from build123d import *

# Parameters (mm, degrees)
BOSS_EXTRUDE1_DEPTH = 30
SKETCH2_R           = 1.5
CUT_EXTRUDE1_DEPTH  = 12
SKETCH3_R           = 1.5
BOSS_EXTRUDE2_DEPTH = 6


with BuildPart() as part:
    # Sketch1 → Boss-Extrude1 (new body)
    with BuildSketch(Plane(origin=(0, 0, 0), x_dir=(1, 0, 0), z_dir=(0, 1, 0))):
        Polygon((3.175426481, 0), (1.58771324, 2.75), (-1.58771324, 2.75), (-3.175426481, 0), (-1.58771324, -2.75), (1.58771324, -2.75), align=None)
    extrude(amount=BOSS_EXTRUDE1_DEPTH)

    # Sketch2 → Cut-Extrude1 (cut)
    with BuildSketch(Plane(origin=(0, 30, 0), x_dir=(1, 0, 0), z_dir=(0, 1, 0))):
        with Locations(Location((0, 0, 0), (0, 0, 270))):
            Circle(SKETCH2_R)
    extrude(amount=-CUT_EXTRUDE1_DEPTH, mode=Mode.SUBTRACT)

    # Sketch3 → Boss-Extrude2 (add)
    with BuildSketch(Plane(origin=(0, 0, 0), x_dir=(-1, 0, 0), z_dir=(0, -1, 0))):
        with Locations(Location((0, 0, 0), (0, 0, 270))):
            Circle(SKETCH3_R)
    extrude(amount=BOSS_EXTRUDE2_DEPTH)


solid = part.part
CAD build for the part. Positions are in the model's coordinates, mm. A direction names the side the tool comes from. Give positions to 0.01 mm unless a question says otherwise; leave off trailing zeros. Loops run counter-clockwise (first coordinate to the right, second up) from the corner with the lowest first, then second, coordinate; pieces in that order, holes last. Notation, with made-up numbers: M 44,52 L 95,52 A25 ccw 95,68 Z; hole C 49,-28.5 d11. An arc over 180 degrees is marked long. Answer in a Markdown table with one row per item. Add a question column.
Item 1: Tool access for faces 1 (the face through (1.4, 0, -1.3)), 2 (the face through (-2.39, 14.79, 1.36)), 3 (the face through (0.45, 24.08, 1.43)): list every direction of +Z, -Z, +X, -X, +Y, -Y with a clear straight run to the whole face (end or side of a thin tool).
Item 2: Band-saw the part on B-B on x = 0. Give the cut face in (y, z), then the cut area to 3 significant figures.
Item 3: Band-saw the part on C-C on z = 1.2. Give the cut face in (x, y), then the cut area to 3 significant figures.
Item 4: Probe probe 1 along Z at (x, y) = (-1.25, 26); probe 2 along Y at (x, z) = (1.25, -2.4); probe 3 along Y at (x, z) = (0.5, 0.9). List the from-to ranges inside material, lowest first.
Item 5: Drop a flat-ended pin along its axis: P1, Ø1.5, axis at x = 0, z = 0, coming from the +Y side. Give the stop position or say it passes through.
Item 6: Band-saw the part on A-A on y = 27. Give the cut face in (x, z), then the cut area to 3 significant figures.
Item 7: Band-saw the part on D-D on y = 17. Give the cut face in (x, z), then the cut area to 3 significant figures.
Reply:
| question | item | result |
|---|---|---|
| 1 | face 1 | -Y |
| 1 | face 2 | +Z, -X, +Y, -Y |
| 1 | face 3 | +Y |
| 2 | outline | M -6,-1.5 L 0,-1.5 L 0,-2.75 L 30,-2.75 L 30,-1.5 L 18,-1.5 L 18,1.5 L 30,1.5 L 30,2.75 L 0,2.75 L 0,1.5 L -6,1.5 Z |
| 2 | area | 147 mm^2 |
| 3 | outline | M -2.48,0 L -0.9,0 L -0.9,-6 L 0.9,-6 L 0.9,0 L 2.48,0 L 2.48,30 L 0.9,30 L 0.9,18 L -0.9,18 L -0.9,30 L -2.48,30 Z |
| 3 | area | 138 mm^2 |
| 4 | probe 1 | z = -2.75 to -0.83, 0.83 to 2.75 |
| 4 | probe 2 | y = 0 to 30 |
| 4 | probe 3 | y = -6 to 18 |
| 5 | P1 | stops at y = 18 |
| 6 | outline | M -3.18,0 L -1.59,-2.75 L 1.59,-2.75 L 3.18,0 L 1.59,2.75 L -1.59,2.75 Z; hole C 0,0 d3 |
| 6 | area | 19.1 mm^2 |
| 7 | outline | M -3.18,0 L -1.59,-2.75 L 1.59,-2.75 L 3.18,0 L 1.59,2.75 L -1.59,2.75 Z |
| 7 | area | 26.2 mm^2 |
